Geometry check sheet. Reference: the model listing, model coordinates, mm. A direction names the side the tool comes from. Coordinates: 2 decimals unless noted, no trailing zeros. Loops run counter-clockwise (first coordinate to the right, second up) from the corner with the lowest first, then second, coordinate; pieces in that order, holes last. Notation, with made-up numbers: M -19.75,82 L 0.25,82 A32 cw 0.25,108 Z; hole C 5,43.5 d11. An arc over 180 degrees is marked long. Use CSV: the item, a comma, the result in double quotes.
```python
from build123d import *

# Parameters (mm, degrees)
F1_DEPTH = 15
F2_W     = 20
F2_H     = 10
F3_DEPTH = 9
F4_R     = 2.49999
F5_W     = 14
F5_H     = 7
F6_DEPTH = 10
F7_R     = 1


# Not quite as in the source:
# - a fillet or chamfer is up to 0.001 mm smaller than in the source, because OpenCascade refuses the exact size


with BuildPart() as f1:
    # F0 (on Right) → F1 (new body, symmetric)
    with BuildSketch(Plane.YZ):
        Polygon((15, 12.5), (15, 17.5), (-5, 17.5), (-5, -17.5), (15, -17.5), (15, -12.5), (0, -12.5), (0, 12.5), align=None)
    extrude(amount=F1_DEPTH, both=True)

    # F2 (on face) → F3 (join)
    with BuildSketch(Plane.XY.offset(17.5)):
        with Locations((0, 5)):
            Rectangle(F2_W, F2_H)
    extrude(amount=F3_DEPTH)

    # F4 (radius 2.5 in the source; OpenCascade refuses exactly that, so slightly less here)
    f4_edges = [f1.edges().sort_by_distance(p)[0] for p in [
        (0, 15, 12.5),
        (0, 15, -12.5),
        (0, 15, 17.5),
        (0, 15, -17.5),
        (0, -5, 17.5),
        (0, -5, -17.5),
    ]]
    fillet(f4_edges, radius=F4_R)

    # F5 (on face) → F6 (cut, through all)
    with BuildSketch(Plane.XZ):
        with Locations((0, 21)):
            Rectangle(F5_W, F5_H)
    extrude(amount=-F6_DEPTH, mode=Mode.SUBTRACT)

    # F7
    f7_edges = [f1.edges().sort_by_distance(p)[0] for p in [
        (-7, 5, 17.5),
        (-7, 5, 24.5),
        (7, 5, 17.5),
        (7, 5, 24.5),
        (-10, 5, 17.5),
        (-10, 5, 26.5),
        (10, 5, 26.5),
        (10, 5, 17.5),
    ]]
    fillet(f7_edges, radius=F7_R)


solid = f1.part
```
1. Thickness scan on line 1 (Z direction, x = 0.5, y = 9); line 2 (Z direction, x = -7.5, y = 7); line 3 (Z direction, x = 13.25, y = 2.25). Record the ranges inside material, lowest first. Write a range as [from, to].
The answers:
line 1,"[-17.5, -12.5], [12.5, 17.5], [24.5, 26.5]"
line 2,"[-17.5, -12.5], [12.5, 26.5]"
line 3,"[-17.5, -12.5], [12.5, 17.5]"
2. Gauge pin test, flat ends, axial feed: P1, Ø2.5, axis at y = 6.5, z = 20.5, coming from the +X side; P2, Ø1.5, axis at x = -4, y = -3, coming from the +Z side; P3, Ø4, axis at x = 0, z = -6.5, coming from the +Y side; P4, Ø4.5, axis at x = 2.5, z = 21, coming from the -Y side. Record the tip position at first contact, or that the pin passes through.
The answers:
P1,"x = 10"
P2,"z = 17.5"
P3,"y = 0"
P4,"through"
3. Set-up check for faces 1 (the flat face through (0, 10, 25)), 2 (the cylindrical face through (0, 14, 13)), 3 (the cylindrical face through (-9.715, 5.07, 26.199)), 4 (the flat face through (-7, 5, 21)): record each of +Z, -Z, +X, -X, +Y, -Y from which the full face is reachable in a straight line by a thin tool's end or side.
The answers:
face 1,"+Z, +X, -X, +Y"
face 2,"+X, -X, +Y"
face 3,"+Z, -X, +Y, -Y"
face 4,"+Y, -Y"
4. Release check for a two-part mould opening along Z. For faces 5 (the flat face through (0, 6, -12.5)), 6 (the flat face through (10, 5, 22)), 7 (the cylindrical face through (6.699, 5.07, 24.215)), 8 (the cylindrical face through (-10.301, 5.07, 17.785)) record: +Z half, -Z half, draft (parallel to the pull), parting line (faces both ways), or undercut.
The answers:
face 5,"undercut"
face 6,"draft"
face 7,"undercut"
face 8,"+Z half"
5. Section check A-A, the plane z = 23. Record the cut outline in (x, y).
The answers:
outline,"M -10,0 L -7,0 L -7,10 L -10,10 Z; M 7,0 L 10,0 L 10,10 L 7,10 Z"
6. Section check B-B, the plane y = 6. Record the cut outline in (x, z).
The answers:
outline,"M -15,-17.5 L 15,-17.5 L 15,-12.5 L -15,-12.5 Z; M -15,12.5 L 15,12.5 L 15,17.5 L 11,17.5 A1 cw 10,18.5 L 10,25.5 A1 ccw 9,26.5 L -9,26.5 A1 ccw -10,25.5 L -10,18.5 A1 cw -11,17.5 L -15,17.5 Z; hole M -7,18.5 A1 ccw -6,17.5 L 6,17.5 A1 ccw 7,18.5 L 7,23.5 A1 ccw 6,24.5 L -6,24.5 A1 ccw -7,23.5 Z"
